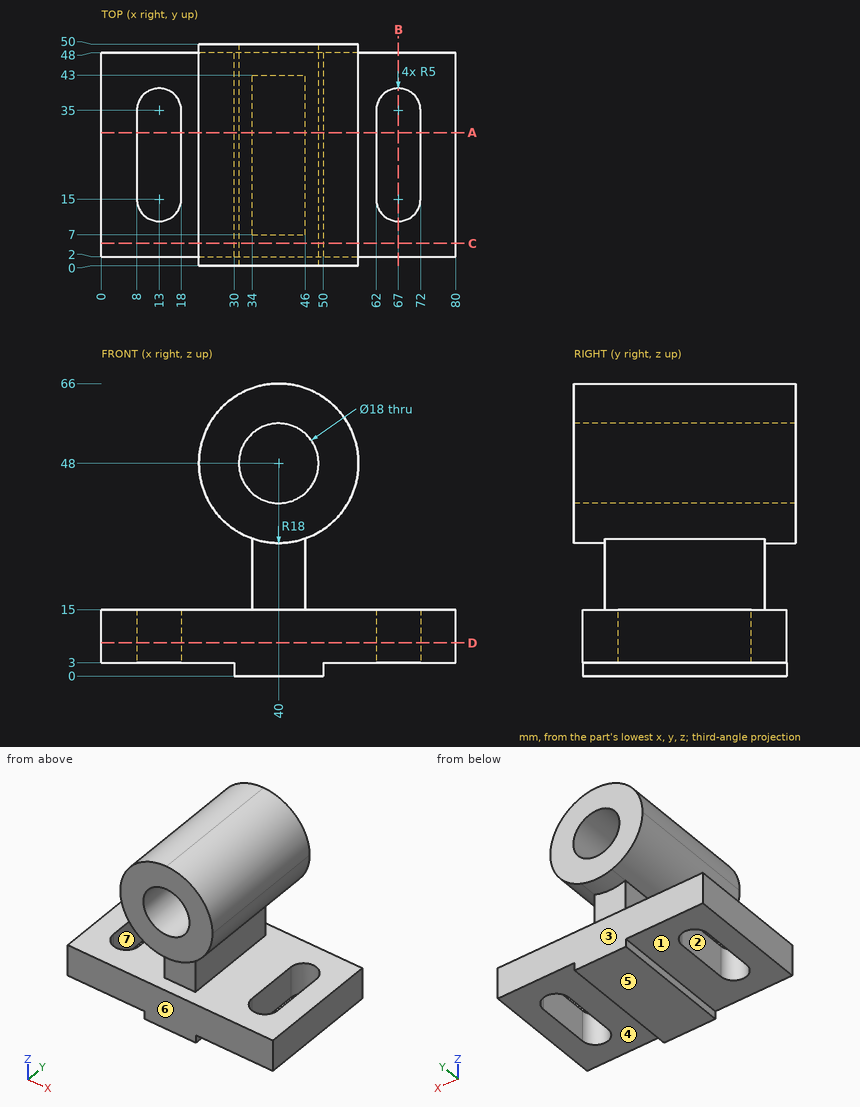
Here's the drawing with two shaded views (mm, measured from the low corner). I have some questions. A direction names the side the tool comes from. Round coordinates to 2 decimals unless told otherwise and drop trailing zeros. Loops run counter-clockwise (first coordinate to the right, second up) from the corner with the lowest first, then second, coordinate; pieces in that order, holes last. Notation, with made-up numbers: M 57.25,-7.5 L 66.25,-7.5 A33 ccw 66.25,31.5 Z; hole C 87,69 d4. An arc over 180 degrees is marked long. Answer as CSV lines item,"result".
1) For pin 1 Ø5 at (x, z) = (35.5, 45.5) entering from +Y; pin 2 Ø16.5 at (x, z) = (34, 7) entering from -Y; pin 3 Ø13 at (x, z) = (40, 21) entering from +Y; pin 4 Ø2 at (x, y) = (16.5, 10.5) entering from -Z, each with a flat end and sliding along its axis, tell me the tip position at first contact or that it passes through.
From the geometry:
pin 1,"through"
pin 2,"y = 2"
pin 3,"y = 48"
pin 4,"z = 3"
2) Imagine slicing it at D-D on z = 7.5. List the corners of the cut face in (x, y) for me, and give its area (3 significant figures).
From the geometry:
outline,"M 0,2 L 80,2 L 80,48 L 0,48 Z; hole M 8,15 A5 ccw 18,15 L 18,35 A5 ccw 8,35 Z; hole M 62,15 A5 ccw 72,15 L 72,35 A5 ccw 62,35 Z"
area,"3,120 mm^2"
3) Imagine slicing it at C-C on y = 5. List the corners of the cut face in (x, z) for me, and give its area (3 significant figures).
From the geometry:
outline,"M 0,3 L 30,3 L 30,0 L 50,0 L 50,3 L 80,3 L 80,15 L 0,15 Z; C 40,48 d36; hole C 40,48 d18"
area,"1,780 mm^2"
4) Imagine slicing it at A-A on y = 30. List the corners of the cut face in (x, z) for me, and give its area (3 significant figures).
From the geometry:
outline,"M 0,3 L 8,3 L 8,15 L 0,15 Z; M 18,3 L 30,3 L 30,0 L 50,0 L 50,3 L 62,3 L 62,15 L 46,15 L 46,31.03 A18 ccw long 34,31.03 L 34,15 L 18,15 Z; M 72,3 L 80,3 L 80,15 L 72,15 Z; hole C 40,48 d18"
area,"1,730 mm^2"
5) Which directions (+Z, -Z, +X, -X, +Y, -Y) give clear straight access to the entire face, cutting with the end or side of a thin tool? Please do the marked faces 1, 2, 3 and 4.
From the geometry:
face 1,"-Z, -X, +Y, -Y"
face 2,"+Z, -Z"
face 3,"-Z, +X, -X, +Y"
face 4,"-Z, +X, +Y, -Y"
6) We'd pull the mould along Y, two halves only. Please class the marked faces 5, 6 and 7: released by +Y, released by -Y, zero draft, split by the parting line, or undercut.
From the geometry:
face 5,"zero draft"
face 6,"released by -Y"
face 7,"undercut"
7) Imagine slicing it at B-B on x = 67. List the corners of the cut face in (y, z) for me, and give its area (3 significant figures).
From the geometry:
outline,"M 2,3 L 10,3 L 10,15 L 2,15 Z; M 40,3 L 48,3 L 48,15 L 40,15 Z"
area,"192 mm^2"
8) If I drill on probe 1 along Z at (x, y) = (40, 21); probe 2 along Z at (x, y) = (68.5, 8); probe 3 along Y at (x, z) = (17, 8), over which ranges is the centre line in solid material (lowest first)?
From the geometry:
probe 1,"0 to 39, 57 to 66"
probe 2,"3 to 15"
probe 3,"2 to 12, 38 to 48"
